CAD build for the part. Positions are in the model's coordinates, mm. Face numbers are marked on the shaded views. Give positions to 0.01 mm unless a question says otherwise; leave off trailing zeros. Write each loop counter-clockwise with the first axis right and the second up, starting at its lowest first coordinate (ties: lowest second). Pieces come first, ordered by that corner, then holes. Notation, with made-up numbers: (41, 36.5) -> (84, 36.5) arc R20 ccw to (84, 69.5) -> close; hole circle Ø10 at (14.25, 38). An arc over 180 degrees is marked (long way). Answer in a Markdown table with one row per item. Add a question column.
```python
from build123d import *

# Parameters (mm, degrees)
ESQUISSE2_R        = 2
ESQUISSE2_R_2      = 13.315
BOSS_EXTRU_1_DEPTH = 5
CONG_1_R           = 5


with BuildPart() as part:
    # Esquisse2 → Boss.-Extru.1 (new body)
    with BuildSketch(Plane.XY):
        with BuildLine():
            Line((-50, 20), (-50, 0))
            Line((-50, 0), (50, 0))
            Line((50, 0), (50, 20))
            ThreePointArc((50, 20), (0, 56.025428048), (-50, 20))
        make_face()
        with Locations((-40, 10)):
            Circle(ESQUISSE2_R, mode=Mode.SUBTRACT)
        with Locations(Location((40, 10, 0), (0, 0, 180))):
            Circle(ESQUISSE2_R, mode=Mode.SUBTRACT)
        with Locations((0, 33.315)):
            Circle(ESQUISSE2_R_2, mode=Mode.SUBTRACT)
    extrude(amount=BOSS_EXTRU_1_DEPTH)

    # Congé1
    cong_1_edges = [part.edges().sort_by_distance(p)[0] for p in [
        (50, 20, 2.5),
        (50, 0, 2.5),
        (-50, 0, 2.5),
        (-50, 20, 2.5),
    ]]
    fillet(cong_1_edges, radius=CONG_1_R)


solid = part.part
```
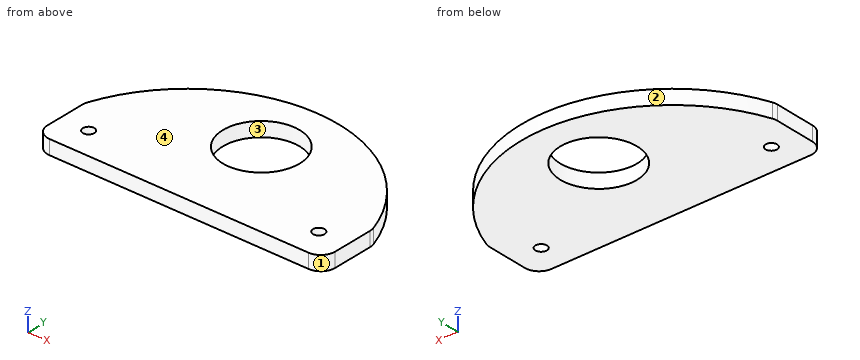
Item 1: Slice it at B-B, the plane y = 22.5. List the corners of the cut face in (x, z).
Item 2: Slice it at A-A, the plane y = 10. List the corners of the cut face in (x, z).
Item 3: Slice it at C-C, the plane x = 40. List the corners of the cut face in (y, z), then the cut area to 3 significant figures.
Item 4: Drop flat-ended pins along their axis: pin 1 Ø2 at (x, z) = (-27.5, 2.5) entering from +Y; pin 2 Ø2 at (x, z) = (-10, 0.5) entering from +Y; pin 3 Ø3 at (x, y) = (-33, 32) entering from -Z; pin 4 Ø2 at (y, z) = (46.5, 2.5) entering from +X. Give the stop position or say it passes through.
Item 5: Slice it at D-D, the plane z = 3.25. List the corners of the cut face in (x, y) (3 decimals).
Item 6: Probe L1, parallel to Y at x = 0, z = 1.7; L2, parallel to X at y = 8.5, z = 1.4; L3, parallel to Y at x = -40, z = 3.75. List the from-to ranges inside material, lowest first. Write a range as from..to.
Item 7: Mould opens along Y. For the marked faces 1, 2, 3 and 4 say: released by +Y, released by -Y, zero draft, split by the parting line, or undercut.
Answer key:
| question | item | result |
|---|---|---|
| 1 | outline | (-49.1, 0) -> (-7.77, 0) -> (-7.77, 5) -> (-49.1, 5) -> close; (7.77, 0) -> (49.1, 0) -> (49.1, 5) -> (7.77, 5) -> close |
| 2 | outline | (-50, 0) -> (-42, 0) -> (-42, 5) -> (-50, 5) -> close; (-38, 0) -> (38, 0) -> (38, 5) -> (-38, 5) -> close; (42, 0) -> (50, 0) -> (50, 5) -> (42, 5) -> close |
| 3 | outline | (0, 0) -> (8, 0) -> (8, 5) -> (0, 5) -> close; (12, 0) -> (37.64, 0) -> (37.64, 5) -> (12, 5) -> close |
| 3 | area | 168 mm² |
| 4 | pin 1 | stops at y = 48.88 |
| 4 | pin 2 | stops at y = 55.25 |
| 4 | pin 3 | stops at z = 0 |
| 4 | pin 4 | stops at x = 31.6 |
| 5 | outline | (-50, 5) arc R5 ccw to (-45, 0) -> (45, 0) arc R5 ccw to (50, 5) -> (50, 19.167) arc R5 ccw to (49.716, 20.828) arc R52.71 ccw to (-49.716, 20.828) arc R5 ccw to (-50, 19.167) -> close; hole circle Ø4 at (-40, 10); hole circle Ø26.63 at (0, 33.315); hole circle Ø4 at (40, 10) |
| 6 | L1 | y = 0..20, 46.63..56.03 |
| 6 | L2 | x = -50..-41.32, -38.68..38.68, 41.32..50 |
| 6 | L3 | y = 0..8, 12..37.64 |
| 7 | face 1 | released by -Y |
| 7 | face 2 | released by +Y |
| 7 | face 3 | undercut |
| 7 | face 4 | zero draft |
